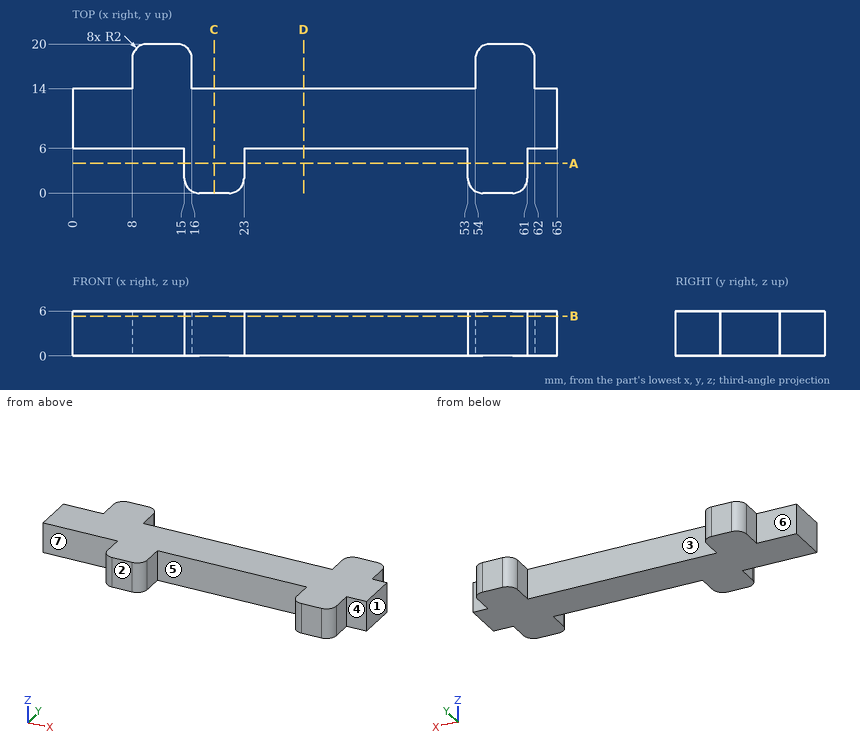
The drawing under review shows one solid part. Ordinate dimensions are in mm from its lowest x, y, z. A direction names the side the tool comes from. Round coordinates to 2 decimals unless told otherwise and drop trailing zeros. Order: outer loops, then holes, each group sorted by start corner. A loop starts at its lowest first (then second) coordinate and runs counter-clockwise, first axis right, second up. Notation, with made-up numbers: (29.5, -9) -> (62.5, -9) arc R20 ccw to (62.5, 13) -> close; hole circle Ø5 at (69, 46.25). An arc over 180 degrees is marked (long way). Use a Markdown table: item, result.
Item 1: Machinability: for the marked faces 4, 5, 6 and 7, which of the approach directions +Z, -Z, +X, -X, +Y, -Y give a long, thin tool a straight path to every point of the face, cutting with its end or side? Answer none if there is none.
Resolved:
| item | result |
|---|---|
| face 4 | +Z, -Z, +X, -Y |
| face 5 | +Z, -Z, -Y |
| face 6 | +Z, -Z, -X, +Y |
| face 7 | +Z, -Z, -X, -Y |
Item 2: For pin 1 (3 mm diameter, centred on y = 3.5, z = 3.5, fed in from +X); pin 2 (1.2 mm diameter, centred on x = 63, z = 1.5, fed in from -Y); pin 3 (2 mm diameter, centred on x = 25.5, y = 16.5, fed in from -Z); pin 4 (1.5 mm diameter, centred on y = 6, z = 2.5, fed in from -X), all flat-tipped, find the tip position at first contact; note any pin that passes through.
Resolved:
| item | result |
|---|---|
| pin 1 | stops at x = 61 |
| pin 2 | stops at y = 6 |
| pin 3 | passes through |
| pin 4 | stops at x = 0 |
Item 3: Take a section at D-D (x = 31). State the section outline as (y, z) points.
Resolved:
| item | result |
|---|---|
| outline | (6, 0) -> (14, 0) -> (14, 6) -> (6, 6) -> close |
Item 4: Take a section at B-B (z = 5.35). State the section outline as (x, y) points.
Resolved:
| item | result |
|---|---|
| outline | (0, 6) -> (15, 6) -> (15, 2) arc R2 ccw to (17, 0) -> (21, 0) arc R2 ccw to (23, 2) -> (23, 6) -> (53, 6) -> (53, 2) arc R2 ccw to (55, 0) -> (59, 0) arc R2 ccw to (61, 2) -> (61, 6) -> (65, 6) -> (65, 14) -> (62, 14) -> (62, 18) arc R2 ccw to (60, 20) -> (56, 20) arc R2 ccw to (54, 18) -> (54, 14) -> (16, 14) -> (16, 18) arc R2 ccw to (14, 20) -> (10, 20) arc R2 ccw to (8, 18) -> (8, 14) -> (0, 14) -> close |
Item 5: Take a section at A-A (y = 4). State the section outline as (x, z) points.
Resolved:
| item | result |
|---|---|
| outline | (15, 0) -> (23, 0) -> (23, 6) -> (15, 6) -> close; (53, 0) -> (61, 0) -> (61, 6) -> (53, 6) -> close |
Item 6: Take a section at C-C (x = 19). State the section outline as (y, z) points, plus the area to 3 significant figures.
Resolved:
| item | result |
|---|---|
| outline | (0, 0) -> (14, 0) -> (14, 6) -> (0, 6) -> close |
| area | 84.0 mm² |
Item 7: Draft analysis for pull direction X (two halves, no side actions). For the marked faces 1, 2 and 3, state which applies: +X half, -X half, draft (parallel to the pull), parting line (faces both ways), or undercut.
Resolved:
| item | result |
|---|---|
| face 1 | +X half |
| face 2 | draft |
| face 3 | undercut |
Item 8: For line 1 along X through (y, z) = (4.5, 5.85); line 2 along X through (y, z) = (17.75, 4.45); line 3 along Y through (x, z) = (6.5, 3.25), list the stretches that pass through material, from the lowest coordinate up. Write a range as [from, to].
Resolved:
| item | result |
|---|---|
| line 1 | x = [15, 23], [53, 61] |
| line 2 | x = [8, 16], [54, 62] |
| line 3 | y = [6, 14] |
